Verification items for the finished model (mm, model axes). Face numbers are marked on the shaded views. A direction names the side the tool comes from. Round coordinates to 2 decimals unless told otherwise and drop trailing zeros. Loops run counter-clockwise (first coordinate to the right, second up) from the corner with the lowest first, then second, coordinate; pieces in that order, holes last.
from build123d import *

# Parameters (mm, degrees)
F1_DEPTH = 75
F2_W     = 10
F2_H     = 12.5
F3_DEPTH = 6.5
F4_DEPTH = 9000
F5_W     = 30
F5_H     = 75
F5_W_2   = 10
F5_H_2   = 50
F6_DEPTH = 10


with BuildPart() as f1:
    # F0 (on Front) → F1 (new body, symmetric)
    with BuildSketch(Plane.XZ):
        with BuildLine():
            Line((100, 13.75), (100, 16.25))
            Line((100, 16.25), (-100, 16.25))
            Line((-100, 16.25), (-100, -16.25))
            Line((-100, -16.25), (70, -16.25))
            ThreePointArc((70, -16.25), (91.2132034356, -7.4632034356), (100, 13.75))
        make_face()
    extrude(amount=F1_DEPTH, both=True)

    # F2 (on face) → F3 (cut)
    with BuildSketch(Plane.XY.offset(16.25)):
        Polygon((87.5, -62.5), (87.5, 62.5), (-87.5, 62.5), (-87.5, 36.7867040902), (-41, 36.7867040902), (-33.5, 36.7867040902), (-33.5, 28.7867040902), (-38.5, 28.7867040902), (-38.5, 31.7867040902), (-46, 31.7867040902), (-87.5, 31.7867040902), (-87.5, 4.8), (-92.5, 1.8), (-100, 1.8), (-100, -1.8), (-92.5, -1.8), (-87.5, -4.8), (-87.5, -31.2132959098), (-38.5, -31.2132959098), (-38.5, -28.2132959098), (-33.5, -28.2132959098), (-33.5, -36.2132959098), (-41, -36.2132959098), (-46, -36.2132959098), (-87.5, -36.2132959098), (-87.5, -62.5), (-77.5, -62.5), align=None)
        Polygon((40, -25), (40, 0), (40, 25), (40, 37.5), (50, 37.5), (50, 25), (50, -25), (50, -37.5), (40, -37.5), align=None, mode=Mode.SUBTRACT)
        with Locations((45, 31.25)):
            Rectangle(F2_W, F2_H)
        with Locations((45, -31.25)):
            Rectangle(F2_W, F2_H)
    extrude(amount=-F3_DEPTH, mode=Mode.SUBTRACT)

    # F4 (cut): a face of the model
    f4_faces = [f1.faces().sort_by_distance(p)[0] for p in [
        (45, 0, 16.25),
    ]]
    extrude(f4_faces, amount=-F4_DEPTH, mode=Mode.SUBTRACT)

    # F5 (on face) → F6 (cut)
    with BuildSketch(Plane(origin=(0, 0, -16.25), x_dir=(1, 0, 0), z_dir=(0, 0, -1))):
        with Locations((85, 0)):
            Rectangle(F5_W, F5_H)
        Polygon((30, 37.5), (30, 0), (30, -37.5), (70, -37.5), (70, 37.5), align=None)
        with Locations((45, 0)):
            Rectangle(F5_W_2, F5_H_2, mode=Mode.SUBTRACT)
    extrude(amount=-F6_DEPTH, mode=Mode.SUBTRACT)


solid = f1.part
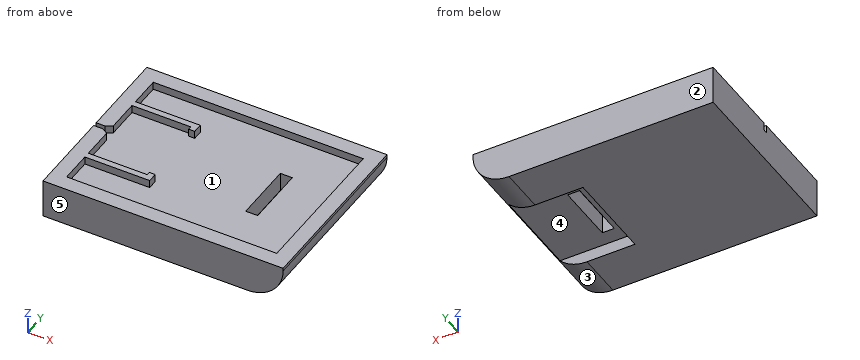
1. Section check B-B (x = 64.5). Enter the section's corners in (y, z), then the cut area to 3 significant figures.
2. Section check D-D (z = -12.5). Enter the section's corners in (x, y).
3. Section check C-C (y = -33.5). Enter the section's corners in (x, z), then the cut area to 3 significant figures.
4. Gauge pin test, flat ends, axial feed: P1, Ø2, axis at y = 34, z = 12, coming from the +X side; P2, Ø2, axis at x = -38.5, y = -55.5, coming from the +Z side; P3, Ø18.5, axis at x = 45.5, y = -3, coming from the -Z side. Record the tip position at first contact, or that the pin passes through.
5. Scan lines: L1, parallel to X at y = 41, z = 14; L2, parallel to Y at x = -17.5, z = 14; L3, parallel to Z at x = -69, y = -10. Record each from-to range of solid material in increasing order.
6. Release check for a two-part mould opening along Y. For the marked faces 1, 2 and 3 record: released by +Y, released by -Y, zero draft, split by the parting line, or undercut.
7. Tool access check on the marked faces 4 and 5. Record the directions out of +Z, -Z, +X, -X, +Y, -Y that give a thin tool (end or side, any length) a straight path to the whole face; none if there is none.
8. Section check A-A (y = 17.5). Enter the section's corners in (x, z).
Taken from the geometry:
1. outline: (-75, -16.25) - (-37.5, -16.25) - (-37.5, -6.25) - (37.5, -6.25) - (37.5, -16.25) - (75, -16.25) - (75, 16.25) - (62.5, 16.25) - (62.5, 9.75) - (-62.5, 9.75) - (-62.5, 16.25) - (-75, 16.25) - close
1. area: 3,310 mm2
2. outline: (-100, -75) - (84.52, -75) - (84.52, -37.5) - (30, -37.5) - (30, 37.5) - (84.52, 37.5) - (84.52, 75) - (-100, 75) - close
3. outline: (-100, -16.25) - (30, -16.25) - (30, -6.25) - (92.36, -6.25) arc R30 ccw to (100, 13.75) - (100, 16.25) - (87.5, 16.25) - (87.5, 9.75) - (-33.5, 9.75) - (-33.5, 16.25) - (-100, 16.25) - close
3. area: 4,970 mm2
4. P1: stops at x = 99.99
4. P2: stops at z = 9.75
4. P3: stops at z = -6.25
5. L1: x = -100 to -87.5, 87.5 to 100
5. L2: y = -75 to -62.5, 62.5 to 75
5. L3: z = -16.25 to 9.75
6. face 1: undercut
6. face 2: released by +Y
6. face 3: zero draft
7. face 4: -Z, +X
7. face 5: +Z, -Z, +X, -X, -Y
8. outline: (-100, -16.25) - (30, -16.25) - (30, -6.25) - (40, -6.25) - (40, 9.75) - (-87.5, 9.75) - (-87.5, 16.25) - (-100, 16.25) - close; (50, -6.25) - (92.36, -6.25) arc R30 ccw to (100, 13.75) - (100, 16.25) - (87.5, 16.25) - (87.5, 9.75) - (50, 9.75) - close
